from build123d import *

# Parameters (mm, degrees)
SKETCH1_W           = 50
SKETCH1_H           = 50
BOSS_EXTRUDE1_DEPTH = 6.35
SKETCH4_R           = 4.5
SKETCH4_W           = 12.5
SKETCH4_H           = 6.35
CUT_EXTRUDE1_DEPTH  = 6.35


with BuildPart() as part:
    # Sketch1 → Boss-Extrude1 (new body)
    with BuildSketch(Plane.XY):
        with Locations((25, 25)):
            Rectangle(SKETCH1_W, SKETCH1_H)
    extrude(amount=BOSS_EXTRUDE1_DEPTH)

    # Sketch4 → Cut-Extrude1 (cut)
    with BuildSketch(Plane.XY.offset(6.35)):
        with Locations((25, 15)):
            Circle(SKETCH4_R)
        with Locations((13.75, 46.825)):
            Rectangle(SKETCH4_W, SKETCH4_H)
        with Locations((36.25, 46.825)):
            Rectangle(SKETCH4_W, SKETCH4_H)
    extrude(amount=-CUT_EXTRUDE1_DEPTH, mode=Mode.SUBTRACT)


solid = part.part
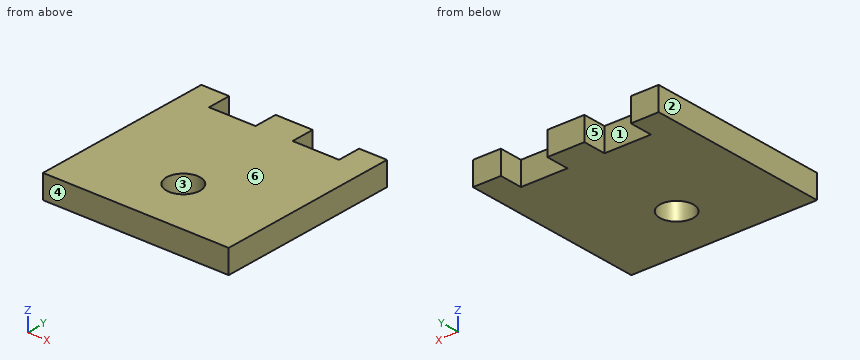
Could you check a few things on this model? Use its own coordinates, in mm. Face numbers are marked on the shaded views. A direction names the side the tool comes from. Coordinates: 2 decimals unless noted, no trailing zeros. Loops run counter-clockwise (first coordinate to the right, second up) from the corner with the lowest first, then second, coordinate; pieces in that order, holes last.
1. For the marked faces 5 and 6, which set-ups out of +Z, -Z, +X, -X, +Y, -Y let a thin tool reach every point of the face, with its end or its side?
2. I need wall thicknesses on L1, parallel to X at y = 47.5, z = 1; L2, parallel to Y at x = 25, z = 3; L3, parallel to Y at x = 35.5, z = 4. Which ranges of each line are inside material? Lowest first, please.
3. Imagine slicing it at D-D (x = 35). Please give me the cut outline in (y, z).
4. Imagine slicing it at C-C (z = 3.25). Please give me the cut outline in (x, y), and give its area (3 significant figures).
5. For P1, Ø3, axis at x = 14, z = 4.5, coming from the +Y side, with a flat end and sliding along its axis, tell me the tip position at first contact or that it passes through.
6. Imagine slicing it at B-B (x = 25). Please give me the cut outline in (y, z), and give its area (3 significant figures).
7. We'd pull the mould along X, two halves only. Please class the marked faces 1, 2, 3 and 4: released by +X, released by -X, zero draft, split by the parting line, or undercut.
8. Imagine slicing it at A-A (y = 15). Please give me the cut outline in (x, z), and give its area (3 significant figures).
Computed values:
1. face 5: +Z, -Z, +Y
1. face 6: +Z, +X, -X, +Y, -Y
2. L1: x = 0 to 7.5, 20 to 30, 42.5 to 50
2. L2: y = 0 to 10.5, 19.5 to 50
2. L3: y = 0 to 43.65
3. outline: (0, 0) - (43.65, 0) - (43.65, 6.35) - (0, 6.35) - close
4. outline: (0, 0) - (50, 0) - (50, 50) - (42.5, 50) - (42.5, 43.65) - (30, 43.65) - (30, 50) - (20, 50) - (20, 43.65) - (7.5, 43.65) - (7.5, 50) - (0, 50) - close; hole circle Ø9 at (25, 15)
4. area: 2,280 mm2
5. P1: stops at y = 43.65
6. outline: (0, 0) - (10.5, 0) - (10.5, 6.35) - (0, 6.35) - close; (19.5, 0) - (50, 0) - (50, 6.35) - (19.5, 6.35) - close
6. area: 260 mm2
7. face 1: undercut
7. face 2: released by -X
7. face 3: undercut
7. face 4: zero draft
8. outline: (0, 0) - (20.5, 0) - (20.5, 6.35) - (0, 6.35) - close; (29.5, 0) - (50, 0) - (50, 6.35) - (29.5, 6.35) - close
8. area: 260 mm2
